Autodesk Inventor part; units mm, degrees
ref_plane "YZ Plane" through (0, 0, 0) normal (1, 0, 0) x (0, 1, 0)
ref_plane "XZ Plane" through (0, 0, 0) normal (0, 1, 0) x (-1, 0, 0)
ref_plane "XY Plane" through (0, 0, 0) normal (0, 0, 1) x (1, 0, 0)
sketch "Sketch1" plane through (0, 0, 0) normal (0, 0, 1) x (1, 0, 0)
  arc A0 (-9.7071, -9.6314) -> (-10, -10.3385) centre (-9, -10.3385) ccw
  line L0 (-10, -10.3385) -> (-10, -13)
  line L1 (-10, -13) -> (-9, -14)
  line L2 (-9, -14) -> (9, -14)
  line L3 (9, -14) -> (10, -13)
  line L4 (10, -13) -> (10, -10.3385)
  arc A1 (10, -10.3385) -> (9.7071, -9.6314) centre (9, -10.3385) ccw
  line L5 (9.7071, -9.6314) -> (6.8929, -6.8172)
  arc A2 (6.6, -6.1101) -> (6.8929, -6.8172) centre (7.6, -6.1101) ccw
  line L6 (6.6, -6.1101) -> (6.6, -4.5499)
  arc A3 (6.8929, -3.8428) -> (6.6, -4.5499) centre (7.6, -4.5499) ccw
  line L7 (6.8929, -3.8428) -> (7.6302, -3.1056)
  arc A4 (7.6302, -3.1056) -> (7.8468, -2.7675) centre (7.3529, -2.6895) ccw
  arc A5 (9.4318, -1.1825) -> (7.8468, -2.7675) centre (9.8106, -3.1463) ccw
  arc A6 (9.4318, -1.1825) -> (9.6906, -1.0451) centre (9.3371, -0.6915) ccw
  line L8 (9.6906, -1.0451) -> (9.8536, -0.8822)
  arc A7 (9.8536, -0.8822) -> (10, -0.5286) centre (9.5, -0.5286) ccw
  line L9 (10, -0.5286) -> (10, 0.5286)
  arc A8 (10, 0.5286) -> (9.8536, 0.8822) centre (9.5, 0.5286) ccw
  line L10 (9.8536, 0.8822) -> (9.6906, 1.0451)
  arc A9 (9.6906, 1.0451) -> (9.4224, 1.1941) centre (9.3254, 0.7036) ccw
  arc A10 (7.8482, 2.768) -> (9.4224, 1.1941) centre (9.8101, 3.1561) ccw
  arc A11 (7.8482, 2.768) -> (7.6325, 3.1032) centre (7.3547, 2.6875) ccw
  line L11 (7.6325, 3.1032) -> (7.2357, 3.5)
  line L12 (7.2357, 3.5) -> (-7.2357, 3.5)
  line L13 (-7.2357, 3.5) -> (-7.6325, 3.1032)
  arc A12 (-7.6325, 3.1032) -> (-7.8482, 2.768) centre (-7.3547, 2.6875) ccw
  arc A13 (-9.4224, 1.1941) -> (-7.8482, 2.768) centre (-9.8101, 3.1561) ccw
  arc A14 (-9.4224, 1.1941) -> (-9.6906, 1.0451) centre (-9.3254, 0.7036) ccw
  line L14 (-9.6906, 1.0451) -> (-9.8536, 0.8822)
  arc A15 (-9.8536, 0.8822) -> (-10, 0.5286) centre (-9.5, 0.5286) ccw
  line L15 (-10, 0.5286) -> (-10, -0.5286)
  arc A16 (-10, -0.5286) -> (-9.8536, -0.8822) centre (-9.5, -0.5286) ccw
  line L16 (-9.8536, -0.8822) -> (-9.6906, -1.0451)
  arc A17 (-9.6906, -1.0451) -> (-9.4318, -1.1825) centre (-9.3371, -0.6915) ccw
  arc A18 (-7.8468, -2.7675) -> (-9.4318, -1.1825) centre (-9.8106, -3.1463) ccw
  arc A19 (-7.8468, -2.7675) -> (-7.6302, -3.1056) centre (-7.3529, -2.6895) ccw
  line L17 (-7.6302, -3.1056) -> (-6.8929, -3.8428)
  arc A20 (-6.6, -4.5499) -> (-6.8929, -3.8428) centre (-7.6, -4.5499) ccw
  line L18 (-6.6, -4.5499) -> (-6.6, -6.1101)
  arc A21 (-6.8929, -6.8172) -> (-6.6, -6.1101) centre (-7.6, -6.1101) ccw
  line L19 (-6.8929, -6.8172) -> (-9.7071, -9.6314)
  point P0 (0, 0)
  point P1 (0, 0)
  dimension "d82" = 18
  dimension "d83" = 14.4714
extrude "Extrusion1" add sketch "Sketch1" along normal blind 250
sketch "Sketch2" plane through (-7.2357, 3.5, 250) normal (0, 1, 0) x (1, 0, 0)
  line L0 (14.4714, 250) -> (0, 250)
  line L1 (0, 250) -> (0, 0)
  line L2 (14.4714, 0) -> (0, 0)
  line L3 (14.4714, 250) -> (14.4714, 0)
  circle A0 centre (7.2357, 1480) radius 4.75
  circle A1 centre (7.2357, 1480) radius 3
  circle A2 centre (7.2357, 1420) radius 4.75
  circle A3 centre (7.2357, 1420) radius 3
  circle A4 centre (7.2357, 1360) radius 4.75
  circle A5 centre (7.2357, 1360) radius 3
  circle A6 centre (7.2357, 1300) radius 4.75
  circle A7 centre (7.2357, 1300) radius 3
  circle A8 centre (7.2357, 1240) radius 4.75
  circle A9 centre (7.2357, 1240) radius 3
  circle A10 centre (7.2357, 1180) radius 4.75
  circle A11 centre (7.2357, 1180) radius 3
  circle A12 centre (7.2357, 1120) radius 4.75
  circle A13 centre (7.2357, 1120) radius 3
  circle A14 centre (7.2357, 1060) radius 4.75
  circle A15 centre (7.2357, 1060) radius 3
  circle A16 centre (7.2357, 1000) radius 4.75
  circle A17 centre (7.2357, 1000) radius 3
  circle A18 centre (7.2357, 940) radius 4.75
  circle A19 centre (7.2357, 940) radius 3
  circle A20 centre (7.2357, 880) radius 4.75
  circle A21 centre (7.2357, 880) radius 3
  circle A22 centre (7.2357, 820) radius 4.75
  circle A23 centre (7.2357, 820) radius 3
  circle A24 centre (7.2357, 760) radius 4.75
  circle A25 centre (7.2357, 760) radius 3
  circle A26 centre (7.2357, 700) radius 4.75
  circle A27 centre (7.2357, 700) radius 3
  circle A28 centre (7.2357, 640) radius 4.75
  circle A29 centre (7.2357, 640) radius 3
  circle A30 centre (7.2357, 580) radius 4.75
  circle A31 centre (7.2357, 580) radius 3
  circle A32 centre (7.2357, 520) radius 4.75
  circle A33 centre (7.2357, 520) radius 3
  circle A34 centre (7.2357, 460) radius 4.75
  circle A35 centre (7.2357, 460) radius 3
  circle A36 centre (7.2357, 400) radius 4.75
  circle A37 centre (7.2357, 400) radius 3
  circle A38 centre (7.2357, 340) radius 4.75
  circle A39 centre (7.2357, 340) radius 3
  circle A40 centre (7.2357, 280) radius 4.75
  circle A41 centre (7.2357, 280) radius 3
  circle A42 centre (7.2357, 220) radius 4.75
  circle A43 centre (7.2357, 220) radius 3
  circle A44 centre (7.2357, 160) radius 4.75
  circle A45 centre (7.2357, 160) radius 3
  circle A46 centre (7.2357, 100) radius 4.75
  circle A47 centre (7.2357, 100) radius 3
  circle A48 centre (7.2357, 40) radius 4.75
  circle A49 centre (7.2357, 40) radius 3
  point P0 (7.2357, 250)
  dimension "d3" = 9.5
  dimension "d4" = 6
  dimension "d6" = 9.5
  dimension "d7" = 6
  dimension "d9" = 9.5
  dimension "d10" = 6
  dimension "d12" = 9.5
  dimension "d13" = 6
  dimension "d15" = 9.5
  dimension "d16" = 6
  dimension "d18" = 9.5
  dimension "d19" = 6
  dimension "d21" = 9.5
  dimension "d22" = 6
  dimension "d24" = 9.5
  dimension "d25" = 6
  dimension "d27" = 9.5
  dimension "d28" = 6
  dimension "d30" = 9.5
  dimension "d31" = 6
  dimension "d33" = 9.5
  dimension "d34" = 6
  dimension "d36" = 9.5
  dimension "d37" = 6
  dimension "d39" = 9.5
  dimension "d40" = 6
  dimension "d42" = 9.5
  dimension "d43" = 6
  dimension "d45" = 9.5
  dimension "d46" = 6
  dimension "d48" = 9.5
  dimension "d49" = 6
  dimension "d51" = 9.5
  dimension "d52" = 6
  dimension "d54" = 9.5
  dimension "d55" = 6
  dimension "d57" = 9.5
  dimension "d58" = 6
  dimension "d60" = 9.5
  dimension "d61" = 6
  dimension "d63" = 9.5
  dimension "d64" = 6
  dimension "d66" = 9.5
  dimension "d67" = 6
  dimension "d69" = 9.5
  dimension "d70" = 6
  dimension "d72" = 9.5
  dimension "d73" = 6
  dimension "d75" = 9.5
  dimension "d76" = 6
extrude "Extrusion2" cut sketch "Sketch2" against normal blind 30 contours A1 | A3 | A5 | A7 | A9 | A11 | A13 | A15 | A17 | A19 | A21 | A23 | A25 | A27 | A29 | A31 | A35 | A37 | A39 | A41 | A43 | A45 | A47 | A49
extrude "Extrusion3" cut sketch "Sketch2" against normal blind 8.4 contours A0 | A2 | A4 | A6 | A8 | A10 | A11 | A12 | A14 | A16 | A18 | A20 | A24 | A26 | A28 | A30 | A32 | A34 | A36 | A38 | A40 | A42 | A44 | A46 | A48
sketch "Sketch3" plane through (0, 0, 250) normal (0, 0, 1) x (1, 0, 0)
  line L0 (9.6906, -1.0451) -> (9.8536, -0.8822)
  arc A0 (9.8536, -0.8822) -> (10, -0.5286) centre (9.5, -0.5286) ccw
  line L1 (10, -0.5286) -> (10, 0.5286)
  arc A1 (10, 0.5286) -> (9.8536, 0.8822) centre (9.5, 0.5286) ccw
  line L2 (9.8536, 0.8822) -> (9.6906, 1.0451)
  arc A2 (9.6906, 1.0451) -> (9.4224, 1.1941) centre (9.3254, 0.7036) ccw
  arc A3 (7.8482, 2.768) -> (9.4224, 1.1941) centre (9.8101, 3.1561) ccw
  arc A4 (7.8482, 2.768) -> (7.6325, 3.1032) centre (7.3547, 2.6875) ccw
  line L3 (7.6325, 3.1032) -> (7.2357, 3.5)
  line L4 (7.2357, 3.5) -> (-7.2357, 3.5)
  line L5 (-7.2357, 3.5) -> (-7.6325, 3.1032)
  arc A5 (-7.6325, 3.1032) -> (-7.8482, 2.768) centre (-7.3547, 2.6875) ccw
  arc A6 (-9.4224, 1.1941) -> (-7.8482, 2.768) centre (-9.8101, 3.1561) ccw
  arc A7 (-9.4224, 1.1941) -> (-9.6906, 1.0451) centre (-9.3254, 0.7036) ccw
  line L6 (-9.6906, 1.0451) -> (-9.8536, 0.8822)
  arc A8 (-9.8536, 0.8822) -> (-10, 0.5286) centre (-9.5, 0.5286) ccw
  line L7 (-10, 0.5286) -> (-10, -0.5286)
  arc A9 (-10, -0.5286) -> (-9.8536, -0.8822) centre (-9.5, -0.5286) ccw
  line L8 (-9.8536, -0.8822) -> (-9.6906, -1.0451)
  arc A10 (-9.6906, -1.0451) -> (-9.4318, -1.1825) centre (-9.3371, -0.6915) ccw
  arc A11 (-7.8468, -2.7675) -> (-9.4318, -1.1825) centre (-9.8106, -3.1463) ccw
  arc A12 (-7.8468, -2.7675) -> (-7.6302, -3.1056) centre (-7.3529, -2.6895) ccw
  line L9 (-7.6302, -3.1056) -> (-6.8929, -3.8428)
  arc A13 (-6.6, -4.5499) -> (-6.8929, -3.8428) centre (-7.6, -4.5499) ccw
  line L10 (-6.6, -4.5499) -> (-6.6, -6.1101)
  arc A14 (-6.8929, -6.8172) -> (-6.6, -6.1101) centre (-7.6, -6.1101) ccw
  line L11 (-6.8929, -6.8172) -> (-9.7071, -9.6314)
  arc A15 (-9.7071, -9.6314) -> (-10, -10.3385) centre (-9, -10.3385) ccw
  line L12 (-10, -10.3385) -> (-10, -13)
  line L13 (-10, -13) -> (-9, -14)
  line L14 (-9, -14) -> (9, -14)
  line L15 (9, -14) -> (10, -13)
  line L16 (10, -13) -> (10, -10.3385)
  arc A16 (10, -10.3385) -> (9.7071, -9.6314) centre (9, -10.3385) ccw
  line L17 (9.7071, -9.6314) -> (6.8929, -6.8172)
  arc A17 (6.6, -6.1101) -> (6.8929, -6.8172) centre (7.6, -6.1101) ccw
  line L18 (6.6, -6.1101) -> (6.6, -4.5499)
  arc A18 (6.8929, -3.8428) -> (6.6, -4.5499) centre (7.6, -4.5499) ccw
  line L19 (6.8929, -3.8428) -> (7.6302, -3.1056)
  arc A19 (7.6302, -3.1056) -> (7.8468, -2.7675) centre (7.3529, -2.6895) ccw
  arc A20 (9.4318, -1.1825) -> (7.8468, -2.7675) centre (9.8106, -3.1463) ccw
  arc A21 (9.4318, -1.1825) -> (9.6906, -1.0451) centre (9.3371, -0.6915) ccw
  line L20 (-4.75, 3.5) -> (4.75, 3.5)
  line L21 (0, 3.5) -> (0, -14)
  point P0 (0, 0)
sketch "Sketch4" plane through (0, 0, 0) normal (0, 0, -1) x (-1, 0, 0)
  line L0 (-9.6906, -1.0451) -> (-9.8536, -0.8822)
  arc A0 (-9.6906, -1.0451) -> (-9.4318, -1.1825) centre (-9.3371, -0.6915) ccw
  arc A1 (-9.4318, -1.1825) -> (-7.8468, -2.7675) centre (-9.8106, -3.1463) ccw
  arc A2 (-7.8468, -2.7675) -> (-7.6302, -3.1056) centre (-7.3529, -2.6895) ccw
  line L1 (-6.8929, -3.8428) -> (-7.6302, -3.1056)
  arc A3 (-6.8929, -3.8428) -> (-6.6, -4.5499) centre (-7.6, -4.5499) ccw
  line L2 (-6.6, -6.1101) -> (-6.6, -4.5499)
  arc A4 (-6.6, -6.1101) -> (-6.8929, -6.8172) centre (-7.6, -6.1101) ccw
  line L3 (-9.7071, -9.6314) -> (-6.8929, -6.8172)
  arc A5 (-9.7071, -9.6314) -> (-10, -10.3385) centre (-9, -10.3385) ccw
  line L4 (-10, -13) -> (-10, -10.3385)
  line L5 (-9, -14) -> (-10, -13)
  line L6 (9, -14) -> (-9, -14)
  line L7 (10, -13) -> (9, -14)
  line L8 (10, -10.3385) -> (10, -13)
  arc A6 (10, -10.3385) -> (9.7071, -9.6314) centre (9, -10.3385) ccw
  line L9 (6.8929, -6.8172) -> (9.7071, -9.6314)
  arc A7 (6.8929, -6.8172) -> (6.6, -6.1101) centre (7.6, -6.1101) ccw
  line L10 (6.6, -4.5499) -> (6.6, -6.1101)
  arc A8 (6.6, -4.5499) -> (6.8929, -3.8428) centre (7.6, -4.5499) ccw
  line L11 (7.6302, -3.1056) -> (6.8929, -3.8428)
  arc A9 (7.6302, -3.1056) -> (7.8468, -2.7675) centre (7.3529, -2.6895) ccw
  arc A10 (7.8468, -2.7675) -> (9.4318, -1.1825) centre (9.8106, -3.1463) ccw
  arc A11 (9.4318, -1.1825) -> (9.6906, -1.0451) centre (9.3371, -0.6915) ccw
  line L12 (9.8536, -0.8822) -> (9.6906, -1.0451)
  arc A12 (9.8536, -0.8822) -> (10, -0.5286) centre (9.5, -0.5286) ccw
  line L13 (10, 0.5286) -> (10, -0.5286)
  arc A13 (10, 0.5286) -> (9.8536, 0.8822) centre (9.5, 0.5286) ccw
  line L14 (9.6906, 1.0451) -> (9.8536, 0.8822)
  arc A14 (9.6906, 1.0451) -> (9.4224, 1.1941) centre (9.3254, 0.7036) ccw
  arc A15 (9.4224, 1.1941) -> (7.8482, 2.768) centre (9.8101, 3.1561) ccw
  arc A16 (7.8482, 2.768) -> (7.6325, 3.1032) centre (7.3547, 2.6875) ccw
  line L15 (7.2357, 3.5) -> (7.6325, 3.1032)
  line L16 (-7.2357, 3.5) -> (7.2357, 3.5)
  line L17 (-7.6325, 3.1032) -> (-7.2357, 3.5)
  arc A17 (-7.6325, 3.1032) -> (-7.8482, 2.768) centre (-7.3547, 2.6875) ccw
  arc A18 (-7.8482, 2.768) -> (-9.4224, 1.1941) centre (-9.8101, 3.1561) ccw
  arc A19 (-9.4224, 1.1941) -> (-9.6906, 1.0451) centre (-9.3254, 0.7036) ccw
  line L18 (-9.8536, 0.8822) -> (-9.6906, 1.0451)
  arc A20 (-9.8536, 0.8822) -> (-10, 0.5286) centre (-9.5, 0.5286) ccw
  line L19 (-10, -0.5286) -> (-10, 0.5286)
  arc A21 (-10, -0.5286) -> (-9.8536, -0.8822) centre (-9.5, -0.5286) ccw
  line L20 (0, 3.5) -> (0, -14)
  point P0 (0, 0)
properties part number "Thanh_truot_20x200"
Geometry: final body of the model. Coordinates: model frame, mm. A direction names the side the tool comes from. Give positions to 0.01 mm unless a question says otherwise; leave off trailing zeros. Answer in a Markdown table with one row per item.
(1) Pin query (flat end, axial travel): pin 1 (7.5 mm diameter, centred on x = 0, z = 90, fed in from +Y); pin 2 (0.8 mm diameter, centred on y = -5.5, z = 150, fed in from -X); pin 3 (10 mm diameter, centred on x = 5.5, y = -3, fed in from -Z); pin 4 (5.5 mm diameter, centred on x = 0, z = 210, fed in from +Y). Return the tip coordinate at first contact, or that it passes through.
Answers below:
| item | result |
|---|---|
| pin 1 | y = -4.9 |
| pin 2 | x = -6.6 |
| pin 3 | z = 0 |
| pin 4 | through |
(2) Draft query along Z for faces 3 (the flat face through (1, -4.9, 213)), 4 (the flat face through (0, -5, 250)), 5 (the flat face through (0, -14, 123)). Return one class per face: +Z half, -Z half, draft (parallel to the pull), parting line (faces both ways), or undercut.
Answers below:
| item | result |
|---|---|
| face 3 | undercut |
| face 4 | +Z half |
| face 5 | draft |
(3) Set-up query: faces 1 (the cylindrical face through (-0.65, -9.39, 32.93)), 2 (the flat face through (1, -4.9, 153)). Return all of +Z, -Z, +X, -X, +Y, -Y with unobstructed straight access to the full face (end or side cutting, diameter ignored); none if empty.
Answers below:
| item | result |
|---|---|
| face 1 | +Y, -Y |
| face 2 | +Y |
(4) Ray query, line 1 along Z through (x, y) = (0, -7.25); line 2 along Z through (x, y) = (0, 1); line 3 along X through (y, z) = (-10.5, 210). Return the intervals inside material, ascending. Write a range as [from, to].
Answers below:
| item | result |
|---|---|
| line 1 | [0, 27], [33, 87], [93, 147], [153, 207], [213, 250] |
| line 2 | [0, 25.25], [34.75, 85.25], [94.75, 145.25], [154.75, 205.25], [214.75, 250] |
| line 3 | [-10, -3], [3, 10] |
(5) Section query A-A on x = 0. State how many separate pieces and enclosed holes the cut face has, then the cut area to 3 significant figures.
Answers below:
| item | result |
|---|---|
| separate pieces | 5 |
| enclosed holes | 0 |
| area | 3,840 mm^2 |
